Part model, mm, in its own coordinate system. A direction names the side the tool comes from. Give positions to 0.01 mm unless a question says otherwise; leave off trailing zeros. Write each loop counter-clockwise with the first axis right and the second up, starting at its lowest first coordinate (ties: lowest second). Pieces come first, ordered by that corner, then holes. Notation, with made-up numbers: (43.5, 28) - (85.5, 28) arc R12 ccw to (85.5, 33) - close; hole circle Ø2 at (50, 70). An arc over 180 degrees is marked (long way). Answer in a Markdown table with one row per item. Add a question column.
1. Pull direction Y, two halves, no side cores. Call faces 3 (the cylindrical face through (161.068, -21.816, -151.148)), 4 (the flat face through (-5, -25, -152.4)), 5 (the cylindrical face through (161.068, -21.816, 151.112)), 6 (the flat face through (-5, 0, 2)): released by +Y, released by -Y, zero draft, split by the parting line, or undercut.
2. Band-saw the part on C-C on z = -47. Write the cut outline in (x, y), plus the area to 3 significant figures.
3. Band-saw the part on B-B on y = -43. Write the cut outline in (x, z).
4. Band-saw the part on A-A on x = -165.1. Write the cut outline in (y, z), plus the area to 3 significant figures.
5. Band-saw the part on D-D on x = 3.5. Write the cut outline in (y, z), plus the area to 3 significant figures.
6. Which spindle directions (+Z, -Z, +X, -X, +Y, -Y) get a long thin tool onto all of the face, cutting with end or side? Do faces 1 (the flat face through (201.405, -25, -2)), 2 (the flat face through (-202.455, -26, -2)). Say none if no direction does.
7. Drop a flat-ended pin along its axis: pin 1 Ø4 at (x, z) = (-5.5, -95.5) entering from -Y. Give the stop position or say it passes through.
8. Probe line 1 along Y through (x, z) = (-165, 151); line 2 along Z through (x, y) = (-48.5, -13); line 3 along X through (y, z) = (-33.5, 134). List the from-to ranges inside material, lowest first.
```python
from build123d import *

# Parameters (mm, degrees)
F0_W     = 406.4
F0_H     = 304.8
F1_DEPTH = 50.8
F2_T     = -2.54
F5_D     = 15


with BuildPart() as f1:
    # F0 (on Front) → F1 (new body)
    with BuildSketch(Plane.XZ):
        with Locations((-1.795288, 0)):
            Rectangle(F0_W, F0_H)
    extrude(amount=F1_DEPTH)

    # F2
    f2_openings = [f1.faces().sort_by_distance(p)[0] for p in [
        (-1.795288, -50.8, 0),
    ]]
    offset(amount=F2_T, openings=f2_openings)

    # F5 (through all)
    with Locations(Plane.XY.offset(152.4)):
        with Locations((-165.1, -28.140361), (165.1, -28.140361)):
            Hole(F5_D / 2)


solid = f1.part
```
Values:
| question | item | result |
|---|---|---|
| 1 | face 3 | undercut |
| 1 | face 4 | zero draft |
| 1 | face 5 | undercut |
| 1 | face 6 | released by +Y |
| 2 | outline | (-205, -50.8) - (-202.46, -50.8) - (-202.46, -2.54) - (198.86, -2.54) - (198.86, -50.8) - (201.4, -50.8) - (201.4, 0) - (-205, 0) - close |
| 2 | area | 1,280 mm² |
| 3 | outline | (-205, -152.4) - (201.4, -152.4) - (201.4, 152.4) - (-205, 152.4) - close; hole (-202.46, -149.86) - (198.86, -149.86) - (198.86, 149.86) - (-202.46, 149.86) - close |
| 4 | outline | (-50.8, -152.4) - (-35.64, -152.4) - (-35.64, -149.86) - (-50.8, -149.86) - close; (-50.8, 149.86) - (-35.64, 149.86) - (-35.64, 152.4) - (-50.8, 152.4) - close; (-20.64, -152.4) - (0, -152.4) - (0, 152.4) - (-20.64, 152.4) - (-20.64, 149.86) - (-2.54, 149.86) - (-2.54, -149.86) - (-20.64, -149.86) - close |
| 4 | area | 943 mm² |
| 5 | outline | (-50.8, -152.4) - (0, -152.4) - (0, 152.4) - (-50.8, 152.4) - (-50.8, 149.86) - (-2.54, 149.86) - (-2.54, -149.86) - (-50.8, -149.86) - close |
| 5 | area | 1,020 mm² |
| 6 | face 1 | +Z, -Z, +X, +Y, -Y |
| 6 | face 2 | -Y |
| 7 | pin 1 | stops at y = -2.54 |
| 8 | line 1 | y = -50.8 to -35.64, -20.64 to 0 |
| 8 | line 2 | z = -152.4 to -149.86, 149.86 to 152.4 |
| 8 | line 3 | x = -205 to -202.46, 198.86 to 201.4 |
